Geometry: final body of the model. Coordinates: model frame, mm. A direction names the side the tool comes from. Round coordinates to 2 decimals unless told otherwise and drop trailing zeros. Write each loop counter-clockwise with the first axis right and the second up, starting at its lowest first coordinate (ties: lowest second). Pieces come first, ordered by that corner, then holes. Notation, with made-up numbers: M 84,73 L 129,73 A15 ccw 129,101 Z; hole C 50.5,58 d8. An arc over 180 degrees is marked long. Use one line per item in the form item = value. Start each with the question number.
Item 1: Ray query, probe 1 along Z at (x, y) = (85.73, 1.25) (3 decimals); probe 2 along Z at (x, y) = (18, 6.5) (1 decimal); probe 3 along X at (y, z) = (8.6, -77.47) (3 decimals). Return the intervals inside material, ascending.
Item 2: Pin query (flat end, axial travel): pin 1 Ø5 at (x, z) = (18.165, 8.335) entering from +Y; pin 2 Ø1 at (y, z) = (4.5, -86.5) entering from -X; pin 3 Ø6 at (x, y) = (88, 13.5) entering from +Z (3 decimals); pin 4 Ø5 at (x, z) = (7, -62) entering from +Y. Return the tip coordinate at first contact, or that it passes through.
Item 3: Pull-direction query (X, two-part tool) for faces 1 (the flat face through (-5.935, 6, -74)), 2 (the cylindrical face through (1.45, 8.07, -0.06)), 3 (the flat face through (91.665, 6, -74)); classes: pulls with the +X half, pulls with the -X half, needs draft (parallel to the pull), parting line crosses it, or undercut.
Item 4: Reachability of faces 4 (the cylindrical face through (6.72, 4.93, -73.46)), 5 (the cylindrical face through (85.44, 3.06, -75.24)), 6 (the flat face through (68, 3.5, -83)), 7 (the flat face through (6, 6, 11.335)), 8 (the flat face through (-2, 13, 4.035)) from +Z, -Z, +X, -X, +Y, -Y: full face, straight path, thin tool, end or side. Return the list, or none.
Item 5: Section query C-C (x = 28). Return loops of the section in (y, z) (3 decimals).
Item 6: Section query D-D (z = -73.66). Return loops of the section in (x, y) (3 decimals), and give its area (3 significant figures).
Item 7: Section query B-B (y = 13). Return loops of the section in (x, z) (3 decimals).
Item 8: Section query A-A (z = -39.5). Return loops of the section in (x, y) (3 decimals).
Autodesk Inventor part; units mm, degrees
ref_plane "YZ Plane" through (0, 0, 0) normal (1, 0, 0) x (0, 1, 0)
ref_plane "XZ Plane" through (0, 0, 0) normal (0, 1, 0) x (-1, 0, 0)
ref_plane "XY Plane" through (0, 0, 0) normal (0, 0, 1) x (1, 0, 0)
sketch "Sketch1" plane through (0, 0, 0) normal (0, 1, 0) x (-1, 0, 0)
  circle A0 centre (0, 0) radius 1.45
  circle A1 centre (0, -73.66) radius 1.45
  circle A2 centre (-85.73, -77.47) radius 1.45
  circle A3 centre (-85.73, 2.54) radius 1.45
  line L0 (7.135, 12.535) -> (-92.865, 12.535)
  line L1 (-92.865, 12.535) -> (-92.865, -87.465)
  line L2 (-92.865, -87.465) -> (7.135, -87.465)
  line L3 (7.135, -87.465) -> (7.135, 12.535)
  line L4 (0, 0) -> (7.135, 0)
  line L5 (-85.73, 2.54) -> (-92.865, 2.54)
  line L6 (-85.73, -77.47) -> (-85.73, -87.465)
  line L7 (-85.73, 2.54) -> (-85.73, 12.535)
  point P0 (0, 0)
  dimension "d0" = 73.66
  dimension "d1" = 80.01
  dimension "d2" = 85.73
  dimension "d3" = 2.54
  dimension "d4" = 3.81
  dimension "d6" = 2.9
  dimension "d7" = 100
  dimension "d8" = 100
extrude "Extrusion1" add sketch "Sketch1" along normal blind 10 contours L3 L2 L1 L5 A3 L7 L0 | L7 A3 L5 L1 L0
sketch "Sketch4" plane through (0, 0, 0) normal (0, -1, 0) x (1, 0, 0)
  line L0 (92.865, -87.465) -> (-7.135, -87.465)
  line L1 (92.865, 12.535) -> (92.865, -87.465)
  line L2 (-7.135, 12.535) -> (92.865, 12.535)
  line L3 (-7.135, -87.465) -> (-7.135, 12.535)
  circle A0 centre (85.73, 2.54) radius 1.45
  circle A1 centre (0, 0) radius 1.45
  circle A2 centre (85.73, -77.47) radius 1.45
  circle A3 centre (0, -73.66) radius 1.45
  circle A4 centre (0, 0) radius 2.25
  circle A5 centre (0, -73.66) radius 2.25
  circle A6 centre (85.73, -77.47) radius 2.25
  circle A7 centre (85.73, 2.54) radius 2.25
  point P0 (0, 0)
  dimension "d13" = 4.5
  dimension "d14" = 4.5
  dimension "d15" = 4.5
  dimension "d16" = 4.5
extrude "Extrusion2" cut sketch "Sketch4" against normal blind 6.2 contours A0 | A1 | A2 | A3 | A4 | A5 | A6 | A7
sketch "Sketch5" plane through (0, 0, 0) normal (0, -1, 0) x (1, 0, 0)
  circle A0 centre (85.73, 2.54) radius 2.25
  circle A1 centre (0, 0) radius 2.25
  circle A2 centre (85.73, -77.47) radius 2.25
  circle A3 centre (0, -73.66) radius 2.25
  line L0 (92.865, -87.465) -> (-7.135, -87.465)
  line L1 (92.865, 12.535) -> (92.865, -87.465)
  line L2 (-7.135, 12.535) -> (92.865, 12.535)
  line L3 (-7.135, -87.465) -> (-7.135, 12.535)
  line L4 (-7.135, -87.465) -> (92.865, 12.535)
  line L5 (-7.135, -12.465) -> (-5.935, -12.465)
  line L6 (-5.935, -12.465) -> (-5.935, 11.335)
  line L7 (-5.935, 11.335) -> (17.865, 11.335)
  line L8 (17.865, 11.335) -> (17.865, 12.535)
  line L9 (-7.135, 12.535) -> (92.865, 12.535)
  line L10 (17.865, -86.265) -> (-5.935, -86.265)
  line L11 (-5.935, -62.465) -> (-7.135, -62.465)
  line L12 (-5.935, -86.265) -> (-5.935, -62.465)
  line L13 (17.865, -87.465) -> (17.865, -86.265)
  line L14 (91.665, -62.465) -> (91.665, -86.265)
  line L15 (67.865, -86.265) -> (67.865, -87.465)
  line L16 (91.665, -86.265) -> (67.865, -86.265)
  line L17 (92.865, -62.465) -> (91.665, -62.465)
  line L18 (67.865, 11.335) -> (91.665, 11.335)
  line L19 (91.665, -12.465) -> (92.865, -12.465)
  line L20 (91.665, 11.335) -> (91.665, -12.465)
  line L21 (67.865, 12.535) -> (67.865, 11.335)
  point P0 (0, 0)
  point P1 (42.865, -37.465)
  point P2 (17.865, 12.535)
  point P3 (17.865, -87.465)
  point P4 (-7.135, -62.465)
  point P5 (67.865, -87.465)
  point P6 (92.865, -62.465)
  point P7 (67.865, 12.535)
  point P8 (92.865, -12.465)
  dimension "d19" = 1.2
  dimension "d20" = 1.2
  dimension "d21" = 25
  dimension "d22" = 25
  dimension "d27" = 360
extrude "Extrusion3" cut sketch "Sketch5" along normal through all both and the other way through all contours L18 L21 L2 L4 | L4 L1 L19 L20 | L10 L13 L0 L4 | L4 L3 L11 L12 | L1 L0 L15 L16 L14 L17 | L8 L7 L6 L5 L3 L2
fillet "Fillet1" radius 1 4 edges at (-5.935, 5, -86.265) (91.665, 5, -86.265) (-5.935, 5, 11.335) (91.665, 5, 11.335)
sketch "Sketch6" plane through (0, 10, 0) normal (0, 1, 0) x (1, 0, 0)
  arc A0 (90.665, -11.335) -> (91.665, -10.335) centre (90.665, -10.335) ccw
  line L0 (91.665, -10.335) -> (91.665, 12.465)
  line L1 (91.665, 12.465) -> (92.865, 12.465)
  line L2 (92.865, 12.465) -> (92.865, 62.465)
  line L3 (92.865, 62.465) -> (91.665, 62.465)
  line L4 (91.665, 62.465) -> (91.665, 85.265)
  arc A1 (91.665, 85.265) -> (90.665, 86.265) centre (90.665, 85.265) ccw
  line L5 (90.665, 86.265) -> (67.865, 86.265)
  line L6 (67.865, 86.265) -> (67.865, 87.465)
  line L7 (67.865, 87.465) -> (17.865, 87.465)
  line L8 (17.865, 87.465) -> (17.865, 86.265)
  line L9 (17.865, 86.265) -> (-4.935, 86.265)
  arc A2 (-4.935, 86.265) -> (-5.935, 85.265) centre (-4.935, 85.265) ccw
  line L10 (-5.935, 85.265) -> (-5.935, 62.465)
  line L11 (-5.935, 62.465) -> (-7.135, 62.465)
  line L12 (-7.135, 62.465) -> (-7.135, 12.465)
  line L13 (-7.135, 12.465) -> (-5.935, 12.465)
  line L14 (-5.935, 12.465) -> (-5.935, -10.335)
  arc A3 (-5.935, -10.335) -> (-4.935, -11.335) centre (-4.935, -10.335) ccw
  line L15 (-4.935, -11.335) -> (17.865, -11.335)
  line L16 (17.865, -11.335) -> (17.865, -12.535)
  line L17 (17.865, -12.535) -> (67.865, -12.535)
  line L18 (67.865, -12.535) -> (67.865, -11.335)
  line L19 (67.865, -11.335) -> (90.665, -11.335)
  circle A4 centre (0, 73.66) radius 1.45
  circle A5 centre (85.73, 77.47) radius 1.45
  circle A6 centre (0, 0) radius 1.45
  circle A7 centre (85.73, -2.54) radius 1.45
  line L20 (-5.935, -11.335) -> (1.365, -11.335)
  line L21 (1.365, -11.335) -> (1.365, -4.035)
  line L22 (1.365, -4.035) -> (-5.935, -4.035)
  line L23 (-5.935, -4.035) -> (-5.935, -11.335)
  line L24 (-7.135, 62.465) -> (-7.135, 12.465)
  line L25 (-7.135, 37.465) -> (92.865, 37.465)
  line L26 (92.865, 12.465) -> (92.865, 62.465)
  line L27 (84.365, -11.335) -> (91.665, -11.335)
  line L28 (84.365, -4.035) -> (84.365, -11.335)
  line L29 (91.665, -4.035) -> (84.365, -4.035)
  line L30 (91.665, -11.335) -> (91.665, -4.035)
  line L31 (91.665, 78.965) -> (91.665, 86.265)
  line L32 (84.365, 78.965) -> (91.665, 78.965)
  line L33 (84.365, 86.265) -> (84.365, 78.965)
  line L34 (91.665, 86.265) -> (84.365, 86.265)
  line L35 (1.365, 86.265) -> (-5.935, 86.265)
  line L36 (1.365, 78.965) -> (1.365, 86.265)
  line L37 (-5.935, 78.965) -> (1.365, 78.965)
  line L38 (-5.935, 86.265) -> (-5.935, 78.965)
  point P0 (0, 0)
  point P1 (-5.935, -4.035)
  point P2 (1.365, -11.335)
  point P3 (42.865, 37.465)
  point P4 (-5.935, 78.965)
  point P5 (84.365, 86.265)
  point P6 (85.6076, 78.965)
  point P7 (85.8524, 78.965)
  point P8 (91.665, 78.965)
  point P9 (91.665, -4.035)
  point P10 (84.365, -11.335)
  dimension "d30" = 7.3
  dimension "d31" = 7.3
  dimension "d39" = 360
extrude "Extrusion4" add sketch "Sketch6" along normal blind 6.5 contours L19 L28 L29 L0 A0 | L15 A3 L14 L22 L21 | L32 L33 L5 A1 L4 | L10 A2 L9 L36 L37
chamfer "Chamfer1" distance 1 angle 45 8 edges at (-2.285, 16.5, 4.035) (1.365, 16.5, 7.685) (1.365, 16.5, -82.615) (-2.285, 16.5, -78.965) (84.365, 16.5, -82.615) (88.015, 16.5, -78.965) (88.015, 16.5, 4.035) (84.365, 16.5, 7.685)
sketch "Sketch7" plane through (0, 10, 0) normal (0, 1, 0) x (1, 0, 0)
  circle A0 centre (85.73, -2.54) radius 1.45
  circle A1 centre (0, 0) radius 1.45
  circle A2 centre (85.73, 77.47) radius 1.45
  circle A3 centre (0, 73.66) radius 1.45
  line L0 (1.365, 86.265) -> (1.365, 78.965)
  line L1 (1.365, 78.965) -> (-5.935, 78.965)
  line L2 (-5.935, 78.965) -> (-5.935, 62.465)
  line L3 (-5.935, 62.465) -> (-7.135, 62.465)
  line L4 (-7.135, 62.465) -> (-7.135, 12.465)
  line L5 (-7.135, 12.465) -> (-5.935, 12.465)
  line L6 (-5.935, 12.465) -> (-5.935, -4.035)
  line L7 (-5.935, -4.035) -> (1.365, -4.035)
  line L8 (1.365, -4.035) -> (1.365, -11.335)
  line L9 (1.365, -11.335) -> (17.865, -11.335)
  line L10 (17.865, -11.335) -> (17.865, -12.535)
  line L11 (17.865, -12.535) -> (67.865, -12.535)
  line L12 (67.865, -12.535) -> (67.865, -11.335)
  line L13 (67.865, -11.335) -> (84.365, -11.335)
  line L14 (84.365, -11.335) -> (84.365, -4.035)
  line L15 (84.365, -4.035) -> (91.665, -4.035)
  line L16 (91.665, -4.035) -> (91.665, 12.465)
  line L17 (91.665, 12.465) -> (92.865, 12.465)
  line L18 (92.865, 12.465) -> (92.865, 62.465)
  line L19 (92.865, 62.465) -> (91.665, 62.465)
  line L20 (91.665, 62.465) -> (91.665, 78.965)
  line L21 (91.665, 78.965) -> (84.365, 78.965)
  line L22 (84.365, 78.965) -> (84.365, 86.265)
  line L23 (84.365, 86.265) -> (67.865, 86.265)
  line L24 (67.865, 86.265) -> (67.865, 87.465)
  line L25 (67.865, 87.465) -> (17.865, 87.465)
  line L26 (17.865, 87.465) -> (17.865, 86.265)
  line L27 (17.865, 86.265) -> (1.365, 86.265)
  line L28 (3.865, 76.465) -> (81.865, 76.465)
  line L29 (81.865, 76.465) -> (81.865, -1.535)
  line L30 (81.865, -1.535) -> (3.865, -1.535)
  line L31 (3.865, -1.535) -> (3.865, 76.465)
  point P0 (0, 0)
  dimension "d50" = 11
  dimension "d51" = 11
  dimension "d52" = 11
  dimension "d53" = 11
extrude "Extrusion5" cut sketch "Sketch7" against normal blind 10 contours L28 L29 L30 L31
fillet "Fillet2" radius 10 4 edges at (3.865, 5, -76.465) (81.865, 5, -76.465) (81.865, 5, 1.535) (3.865, 5, 1.535)
sketch "Sketch8" plane through (0, 10, 0) normal (0, 1, 0) x (1, 0, 0)
  line L0 (17.865, -12.535) -> (67.865, -12.535)
  line L1 (42.865, -12.535) -> (42.865, 87.465)
  line L2 (67.865, 87.465) -> (17.865, 87.465)
  line L3 (67.565, 83.265) -> (18.165, 83.265)
  line L4 (18.165, 83.265) -> (18.165, -8.335)
  line L5 (18.165, -8.335) -> (67.565, -8.335)
  line L6 (67.565, -8.335) -> (67.565, 83.265)
  line L7 (67.565, 83.265) -> (18.165, -8.335) construction
  line L8 (18.165, 83.265) -> (67.565, -8.335) construction
  circle A0 centre (18.165, 83.265) radius 2.1
  circle A1 centre (18.165, -8.335) radius 2.1
  circle A2 centre (67.565, -8.335) radius 2.1
  circle A3 centre (67.565, 83.265) radius 2.1
  point P0 (0, 0)
  point P1 (42.865, 37.465)
  dimension "d57" = 49.4
  dimension "d58" = 91.6
  dimension "d59" = 4.2
  dimension "d60" = 4.2
  dimension "d61" = 4.2
  dimension "d62" = 4.2
extrude "Extrusion6" cut sketch "Sketch8" against normal blind 6.5 contours A1 L4 L5 | L5 L4 A1 | A2 L6 L5 | L5 L6 A2 | A3 L6 L3 | L3 L6 A3 | A0 L4 L3 | L3 L4 A0
properties part number "TopSide" material "ABS Plastic"
Working result:
q1.probe_1 = -86.265 to -79.72, -75.22 to 0.29, 4.79 to 11.335
q1.probe_2 = -87.5 to -85.4, -81.2 to -76.5, 1.5 to 6.2, 10.4 to 12.5
q1.probe_3 = -5.935 to 84.28, 87.18 to 91.665
q2.pin_1 = 10
q2.pin_2 = -5.61
q2.pin_3 = 11.335
q2.pin_4 = through
q3.face_1 = pulls with the -X half
q3.face_2 = undercut
q3.face_3 = pulls with the +X half
q4.face_4 = +Y, -Y
q4.face_5 = -Y
q4.face_6 = +Y
q4.face_7 = +Z, -X, +Y, -Y
q4.face_8 = +X, -X, +Y
q5.outline = M 0,-87.465 L 10,-87.465 L 10,-76.465 L 0,-76.465 Z; M 0,1.535 L 10,1.535 L 10,12.535 L 0,12.535 Z
q6.outline = M -5.935,0 L -2.25,0 L -2.25,6.2 L -1.45,6.2 L -1.45,10 L -5.935,10 Z; M 1.45,6.2 L 2.25,6.2 L 2.25,0 L 6.92,0 L 6.92,10 L 1.45,10 Z; M 78.81,0 L 91.665,0 L 91.665,10 L 78.81,10 Z
q6.area = 218 mm²
q7.outline = M -5.935,-85.265 A1 ccw -4.935,-86.265 L 1.365,-86.265 L 1.365,-78.965 L -5.935,-78.965 Z; M -5.935,4.035 L 1.365,4.035 L 1.365,11.335 L -4.935,11.335 A1 ccw -5.935,10.335 Z; M 84.365,-86.265 L 90.665,-86.265 A1 ccw 91.665,-85.265 L 91.665,-78.965 L 84.365,-78.965 Z; M 84.365,4.035 L 91.665,4.035 L 91.665,10.335 A1 ccw 90.665,11.335 L 84.365,11.335 Z
q8.outline = M -7.135,0 L 3.865,0 L 3.865,10 L -7.135,10 Z; M 81.865,0 L 92.865,0 L 92.865,10 L 81.865,10 Z
